Part model, mm, in its own coordinate system. Give positions to 0.01 mm unless a question says otherwise; leave off trailing zeros. Write each loop counter-clockwise with the first axis right and the second up, starting at its lowest first coordinate (ties: lowest second). Pieces come first, ordered by that corner, then holes. Notation, with made-up numbers: (31.5, 23.5) - (75.5, 23.5) arc R20 ccw to (75.5, 40.5) - close; hole circle Ø9 at (14, 2.5). An arc over 180 degrees is marked (long way). Answer in a Markdown table with one row per item. Add a question column.
1. Band-saw the part on A-A on y = -2. Write the cut outline in (x, z).
2. Probe line 1 along X through (y, z) = (5.5, 1.05); line 2 along X through (y, z) = (-24, 0.65); line 3 along Y through (x, z) = (41, 1.2). List the from-to ranges inside material, lowest first.
3. Drop flat-ended pins along their axis: pin 1 Ø0.6 at (y, z) = (0, 1) entering from -X; pin 2 Ø0.6 at (y, z) = (0, 1) entering from +X; pin 3 Ø0.6 at (x, z) = (43.5, 0.5) entering from -Y. Give the stop position or say it passes through.
```python
from build123d import *

# Parameters (mm, degrees)
F1_DEPTH = 1.27


with BuildPart() as f1:
    # F0 (on Top) → F1 (new body)
    with BuildSketch(Plane.XY):
        with BuildLine():
            ThreePointArc((44.196, 22.86), (42.708102, 26.452102), (39.116, 27.94))
            Line((39.116, 27.94), (-39.116, 27.94))
            ThreePointArc((-39.116, 27.94), (-42.708102, 26.452102), (-44.196, 22.86))
            Line((-44.196, 22.86), (-44.196, 6.8072))
            Line((-44.196, 6.8072), (-43.4975, 6.8072))
            Line((-43.4975, 6.8072), (-42.799, 6.8072))
            Line((-42.799, 6.8072), (-42.6085, 6.8072))
            Line((-42.6085, 6.8072), (-42.6085, -6.8072))
            Line((-42.6085, -6.8072), (-42.799, -6.8072))
            Line((-42.799, -6.8072), (-43.4975, -6.8072))
            Line((-43.4975, -6.8072), (-44.196, -6.8072))
            Line((-44.196, -6.8072), (-44.196, -22.86))
            ThreePointArc((-44.196, -22.86), (-42.708102, -26.452102), (-39.116, -27.94))
            Line((-39.116, -27.94), (39.116, -27.94))
            ThreePointArc((39.116, -27.94), (42.708102, -26.452102), (44.196, -22.86))
            Line((44.196, -22.86), (44.196, -6.8072))
            Line((44.196, -6.8072), (43.4975, -6.8072))
            Line((43.4975, -6.8072), (42.799, -6.8072))
            Line((42.799, -6.8072), (42.6085, -6.8072))
            Line((42.6085, -6.8072), (42.6085, 6.8072))
            Line((42.6085, 6.8072), (42.799, 6.8072))
            Line((42.799, 6.8072), (43.4975, 6.8072))
            Line((43.4975, 6.8072), (44.196, 6.8072))
            Line((44.196, 6.8072), (44.196, 22.86))
        make_face()
    extrude(amount=F1_DEPTH)


solid = f1.part
```
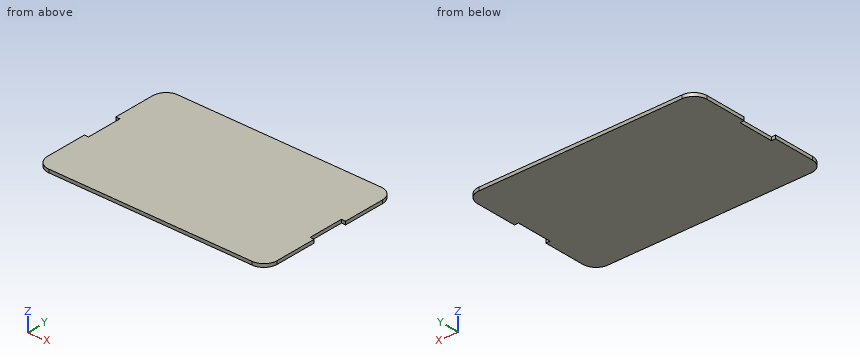
Values:
| question | item | result |
|---|---|---|
| 1 | outline | (-42.61, 0) - (42.61, 0) - (42.61, 1.27) - (-42.61, 1.27) - close |
| 2 | line 1 | x = -42.61 to 42.61 |
| 2 | line 2 | x = -44.07 to 44.07 |
| 2 | line 3 | y = -27.58 to 27.58 |
| 3 | pin 1 | stops at x = -42.61 |
| 3 | pin 2 | stops at x = 42.61 |
| 3 | pin 3 | stops at y = -25.88 |
